Source: CAD feature listing. Evaluate the final solid. Frame: model axes, mm. A direction names the side the tool comes from. Give positions to 0.01 mm unless a question says otherwise; leave off trailing zeros. Loops run counter-clockwise (first coordinate to the right, second up) from the corner with the lowest first, then second, coordinate; pieces in that order, holes last. Notation, with made-up numbers: (70, -28.75) -> (94, -28.75) arc R18 ccw to (94, -10.75) -> close; hole circle Ø6 at (51.25, -36.5). An arc over 180 degrees is marked (long way). Answer as a JSON object with one key per item and string values. Group by question number.
from build123d import *

# Parameters (mm, degrees)
SKETCH1_W           = 165.1
SKETCH1_H           = 101.6
BOSS_EXTRUDE1_DEPTH = 19.05
SKETCH2_W           = 76.2
SKETCH2_H           = 76.2
CUT_EXTRUDE1_DEPTH  = 99.782817332
SKETCH3_R           = 3.175
CUT_EXTRUDE2_DEPTH  = 15.875


with BuildPart() as part:
    # Sketch1 → Boss-Extrude1 (new body)
    with BuildSketch(Plane(origin=(0, 0, 0), x_dir=(1, 0, 0), z_dir=(0, 1, 0))):
        Rectangle(SKETCH1_W, SKETCH1_H)
    extrude(amount=BOSS_EXTRUDE1_DEPTH)

    # Sketch2 → Cut-Extrude1 (cut, through all)
    with BuildSketch(Plane(origin=(0, 19.05, 0), x_dir=(1, 0, 0), z_dir=(0, 1, 0))):
        with Locations((0, 12.7)):
            Rectangle(SKETCH2_W, SKETCH2_H)
    extrude(amount=-CUT_EXTRUDE1_DEPTH, mode=Mode.SUBTRACT)

    # Sketch3 → Cut-Extrude2 (cut)
    with BuildSketch(Plane(origin=(0, 19.05, 0), x_dir=(1, 0, 0), z_dir=(0, 1, 0))):
        with Locations(Location((-60.325, 0, 0), (0, 0, 270))):
            Circle(SKETCH3_R)
        with Locations(Location((60.325, 0, 0), (0, 0, 270))):
            Circle(SKETCH3_R)
    extrude(amount=-CUT_EXTRUDE2_DEPTH, mode=Mode.SUBTRACT)


solid = part.part
(1) Material intervals for line 1 (X direction, y = 7, z = 0); line 2 (X direction, y = 5.75, z = -31); line 3 (Z direction, x = -2, y = 7.5), sorted ascending. Write a range as from..to.
(2) Section query D-D on x = -15. Return the cut outline in (y, z), plus the area to 3 significant figures.
(3) Mould query, pull axis Z, two halves, no side actions, for faces 4 (the face through (-82.55, 9, 1)), 5 (the face through (-1, 10, 25.4)), 6 (the face through (-57.177, 11.224, -0.413)). Classes: pulls with the +Z half, pulls with the -Z half, needs draft (parallel to the pull), parting line crosses it, or undercut.
(4) Section query A-A on z = 0. Return the cut outline in (x, y) (3 decimals), plus the area to 3 significant figures.
(5) First-contact query: pin 1 (8.5 mm diameter, centred on x = 60.325, z = 0, fed in from +Y). Flat tip, straight axial feed; report the tip coordinate or a pass-through.
(6) Section query B-B on z = -14.5. Return the cut outline in (x, y).
(7) Section query C-C on y = 16. Return the cut outline in (x, z) (3 decimals), plus the area to 3 significant figures.
(8) Access query for faces 1 (the face through (-38.1, 10, -12)), 2 (the face through (60, 3.175, 0)), 3 (the face through (-61, 9, -50.8)). Directions: +Z, -Z, +X, -X, +Y, -Y. A direction counts if a zero-diameter tool reaches every point of the face in a straight line with its end or side. Return the directions, or none.
Result:
{
 "1": {"line 1": "-82.55..-63.5, -57.15..-38.1, 38.1..57.15, 63.5..82.55", "line 2": "-82.55..-38.1, 38.1..82.55", "line 3": "25.4..50.8"},
 "2": {"outline": "(0, 25.4) -> (19.05, 25.4) -> (19.05, 50.8) -> (0, 50.8) -> close", "area": "484 mm²"},
 "3": {"face 4": "needs draft", "face 5": "pulls with the -Z half", "face 6": "undercut"},
 "4": {"outline": "(-82.55, 0) -> (-38.1, 0) -> (-38.1, 19.05) -> (-57.15, 19.05) -> (-57.15, 3.175) -> (-63.5, 3.175) -> (-63.5, 19.05) -> (-82.55, 19.05) -> close; (38.1, 0) -> (82.55, 0) -> (82.55, 19.05) -> (63.5, 19.05) -> (63.5, 3.175) -> (57.15, 3.175) -> (57.15, 19.05) -> (38.1, 19.05) -> close", "area": "1,490 mm²"},
 "5": {"pin 1": "y = 19.05"},
 "6": {"outline": "(-82.55, 0) -> (-38.1, 0) -> (-38.1, 19.05) -> (-82.55, 19.05) -> close; (38.1, 0) -> (82.55, 0) -> (82.55, 19.05) -> (38.1, 19.05) -> close"},
 "7": {"outline": "(-82.55, -50.8) -> (-38.1, -50.8) -> (-38.1, 25.4) -> (38.1, 25.4) -> (38.1, -50.8) -> (82.55, -50.8) -> (82.55, 50.8) -> (-82.55, 50.8) -> close; hole circle Ø6.35 at (-60.325, 0); hole circle Ø6.35 at (60.325, 0)", "area": "10,900 mm²"},
 "8": {"face 1": "-Z, +Y, -Y", "face 2": "+Y", "face 3": "-Z, +X, -X, +Y, -Y"}
}
